Verification items for this drawing (mm, ordinates from the low corner). Give positions to 0.01 mm unless a question says otherwise; leave off trailing zeros. Order: outer loops, then holes, each group sorted by start corner. A loop starts at its lowest first (then second) coordinate and runs counter-clockwise, first axis right, second up.
(1) Sectioned sample at A-A on x = 5. Record the cut outline in (y, z).
(2) Sectioned sample at C-C on y = 2. Count the separate pieces of the cut face and the enclosed holes in it, plus the area to 3 significant figures.
(3) Sectioned sample at B-B on z = 25. Record the cut outline in (x, y).
(4) Scan lines: L1, parallel to X at y = 3, z = 154; L2, parallel to Z at x = 114, y = 4.5; L3, parallel to Z at x = 140, y = 3. Record each from-to range of solid material in increasing order.
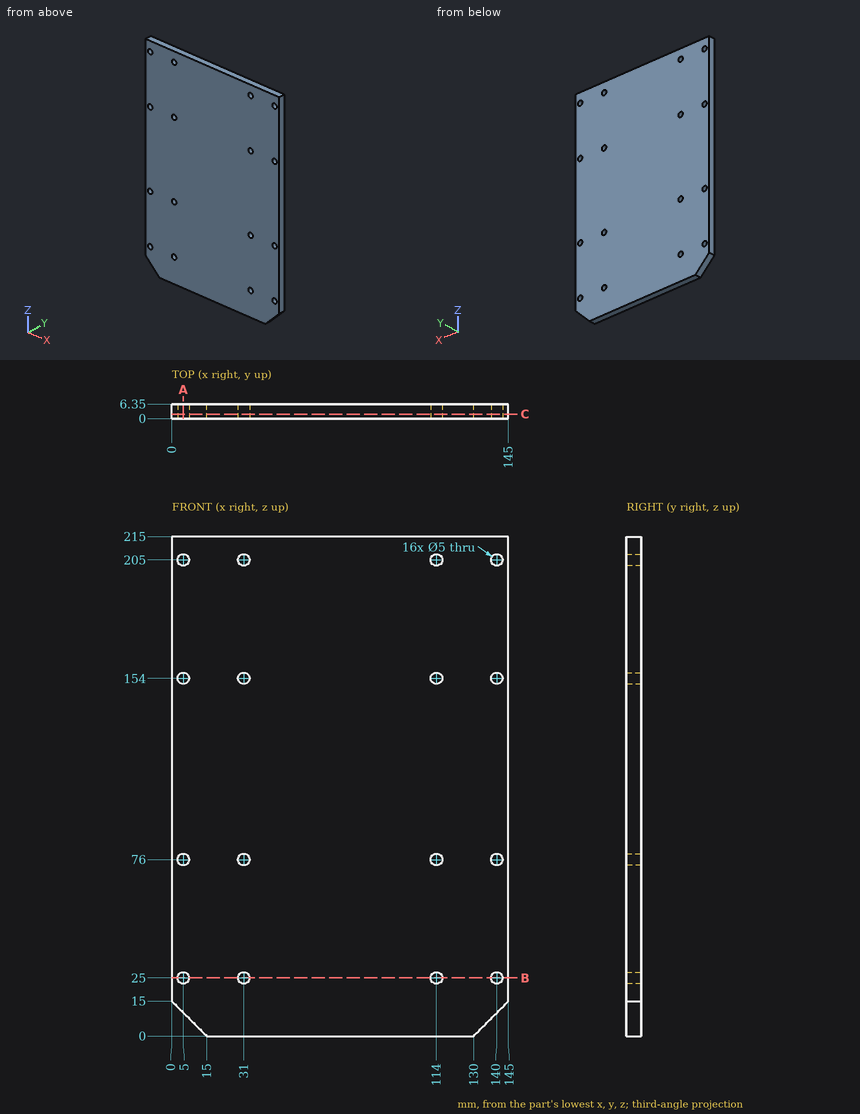
Ans:
1. outline: (0, 10) - (6.35, 10) - (6.35, 22.5) - (0, 22.5) - close; (0, 27.5) - (6.35, 27.5) - (6.35, 73.5) - (0, 73.5) - close; (0, 78.5) - (6.35, 78.5) - (6.35, 151.5) - (0, 151.5) - close; (0, 156.5) - (6.35, 156.5) - (6.35, 202.5) - (0, 202.5) - close; (0, 207.5) - (6.35, 207.5) - (6.35, 215) - (0, 215) - close
2. separate pieces: 1
2. enclosed holes: 16
2. area: 30,600 mm2
3. outline: (0, 0) - (2.5, 0) - (2.5, 6.35) - (0, 6.35) - close; (7.5, 0) - (28.5, 0) - (28.5, 6.35) - (7.5, 6.35) - close; (33.5, 0) - (111.5, 0) - (111.5, 6.35) - (33.5, 6.35) - close; (116.5, 0) - (137.5, 0) - (137.5, 6.35) - (116.5, 6.35) - close; (142.5, 0) - (145, 0) - (145, 6.35) - (142.5, 6.35) - close
4. L1: x = 0 to 2.5, 7.5 to 28.5, 33.5 to 111.5, 116.5 to 137.5, 142.5 to 145
4. L2: z = 0 to 22.5, 27.5 to 73.5, 78.5 to 151.5, 156.5 to 202.5, 207.5 to 215
4. L3: z = 10 to 22.5, 27.5 to 73.5, 78.5 to 151.5, 156.5 to 202.5, 207.5 to 215
